The listing builds one solid part. Answer for the finished solid, in the listing's coordinates (mm). A direction names the side the tool comes from. Give positions to 0.01 mm unless a question says otherwise; leave off trailing zeros. Loops run counter-clockwise (first coordinate to the right, second up) from the corner with the lowest first, then second, coordinate; pieces in that order, holes last.
Item 1: A tool of negligible diameter and unlimited length cuts with its end or side. For faces 1 (the face through (6, 3.5, 4.9)), 2 (the face through (5.51, 2.52, 33.33)), 3 (the face through (-7, 2, 10)), from which of +Z, -Z, +X, -X, +Y, -Y can it reach the whole face along a straight path? Write none if from no direction.
Item 2: Section C-C, the plane z = 4.5 is taken. Give the vertices of the cut face in (x, y), and give its area (3 significant figures).
Item 3: The mould has two halves that part along X. Classify faces 4 (the face through (0, 2, 0)), 5 (the face through (-6, 3.5, 4.9)), 6 (the face through (0.969, 1.972, 25.137)): pulls with the +X half, pulls with the -X half, needs draft (parallel to the pull), parting line crosses it, or undercut.
Item 4: Section A-A, the plane y = 1.6 is taken. Give the vertices of the cut face in (x, z).
Item 5: Section B-B, the plane x = 0 is taken. Give the vertices of the cut face in (y, z).
Item 6: Consider line 1 along Z through (x, y) = (0, 2.55); line 2 along X through (y, z) = (3.45, 6); line 3 along X through (y, z) = (2.5, 25.5). Determine where each line is inside the solid, lowest interval first.
Item 7: Each of these flat-tipped pins is pushed along its axis until it touches: pin 1 Ø2 at (x, z) = (3.5, 6.5) entering from -Y; pin 2 Ø1.5 at (x, y) = (-7, 1) entering from +Z; pin 3 Ø0.5 at (y, z) = (3.5, 5.5) entering from +X; pin 4 Ø2 at (x, y) = (-8, 1) entering from -Z. Where does it stop, or does it pass through?
from build123d import *

# Parameters (mm, degrees)
BOSS_EXTRU_1_DEPTH      = 10
ESQUISSE2_W             = 20
ESQUISSE2_H             = 4
BOSS_EXTRU_2_DEPTH      = 24
ESQUISSE3_R             = 2.1
ENL_V_MAT_EXTRU_1_DEPTH = 5
CHANFREIN1_SIZE         = 10
CHANFREIN1_SIZE2        = 4
CHANFREIN1_PART_2_SIZE  = 10
CHANFREIN1_PART_2_SIZE2 = 4
CONG_1_R                = 4
CONG_2_R                = 1


with BuildPart() as part:
    # Esquisse1 → Boss.-Extru.1 (new body)
    with BuildSketch(Plane.XY):
        Polygon((-3, 0), (3, 0), (6, 3), (6, 4), (-6, 4), (-6, 3), align=None)
    extrude(amount=BOSS_EXTRU_1_DEPTH)

    # Esquisse2 → Boss.-Extru.2 (add)
    with BuildSketch(Plane.XY.offset(10)):
        with Locations((0, 2)):
            Rectangle(ESQUISSE2_W, ESQUISSE2_H)
    extrude(amount=BOSS_EXTRU_2_DEPTH)

    # Esquisse3 → Enlèv. mat.-Extru.1 (cut, through all)
    with BuildSketch(Plane.XZ):
        with Locations((0, 27)):
            Circle(ESQUISSE3_R)
    extrude(amount=-ENL_V_MAT_EXTRU_1_DEPTH, mode=Mode.SUBTRACT)

    # Chanfrein1
    chanfrein1_edges = [part.edges().sort_by_distance(p)[0] for p in [
        (-10, 2, 34),
    ]]
    chanfrein1_side = [part.faces().sort_by_distance(p)[0] for p in [
        (-10, 2, 22),
    ]]
    chamfer(chanfrein1_edges, length=CHANFREIN1_SIZE, length2=CHANFREIN1_SIZE2, reference=chanfrein1_side[0])

    # Chanfrein1 part 2
    chanfrein1_part_2_edges = [part.edges().sort_by_distance(p)[0] for p in [
        (10, 2, 34),
    ]]
    chanfrein1_part_2_side = [part.faces().sort_by_distance(p)[0] for p in [
        (10, 2, 22),
    ]]
    chamfer(chanfrein1_part_2_edges, length=CHANFREIN1_PART_2_SIZE, length2=CHANFREIN1_PART_2_SIZE2, reference=chanfrein1_part_2_side[0])

    # Congé1
    cong_1_edges = [part.edges().sort_by_distance(p)[0] for p in [
        (-6, 2, 34),
        (6, 2, 34),
        (10, 2, 24),
        (-10, 2, 24),
    ]]
    fillet(cong_1_edges, radius=CONG_1_R)

    # Congé2
    cong_2_edges = [part.edges().sort_by_distance(p)[0] for p in [
        (10, 0, 16.614835193),
        (9.927825547, 0, 23.98610047),
        (8.359840841, 0, 28.100397898),
        (5.534383392, 0, 33.312268922),
        (0, 0, 34),
        (-5.534383392, 0, 33.312268922),
        (-8.359840841, 0, 28.100397898),
        (-9.927825547, 0, 23.98610047),
        (-10, 0, 16.614835193),
    ]]
    fillet(cong_2_edges, radius=CONG_2_R)


solid = part.part
Worked answers:
1. face 1: -Z, +X, +Y, -Y
1. face 2: +Z, +X, +Y, -Y
1. face 3: -Z, -X, -Y
2. outline: (-6, 3) - (-3, 0) - (3, 0) - (6, 3) - (6, 4) - (-6, 4) - close
2. area: 39.0 mm2
3. face 4: needs draft
3. face 5: pulls with the -X half
3. face 6: undercut
4. outline: (-10, 10) - (-4.6, 10) - (-4.6, 0) - (4.6, 0) - (4.6, 10) - (10, 10) - (10, 23.23) arc R4 ccw to (9.71, 24.72) - (7.01, 31.49) arc R4 ccw to (3.29, 34) - (-3.29, 34) arc R4 ccw to (-7.01, 31.49) - (-9.71, 24.72) arc R4 ccw to (-10, 23.23) - close; hole circle Ø4.2 at (0, 27)
5. outline: (0, 0) - (4, 0) - (4, 24.9) - (0, 24.9) - close; (0, 29.1) - (4, 29.1) - (4, 34) - (1, 34) arc R1 ccw to (0, 33) - close
6. line 1: z = 0 to 24.9, 29.1 to 34
6. line 2: x = -6 to 6
6. line 3: x = -9.4 to -1.47, 1.47 to 9.4
7. pin 1: stops at y = 0
7. pin 2: stops at z = 32.69
7. pin 3: stops at x = 6
7. pin 4: stops at z = 10
